Input: part model. Units: mm. Frame: model coordinates. A direction names the side the tool comes from. Round coordinates to 2 decimals unless told otherwise and drop trailing zeros. Write each loop counter-clockwise with the first axis right and the second up, starting at its lowest first coordinate (ties: lowest second). Pieces come first, ordered by that corner, then holes. Notation, with made-up numbers: (39, -30.5) - (91, -30.5) arc R27 cw to (91, -10.5) - close; hole circle Ø5 at (-27.75, 43). An arc over 180 degrees is marked (long way). One line per item, written item: value. Start each with the question number.
```python
from build123d import *

# Parameters (mm, degrees)
BOSS_EXTRUDE1_DEPTH = 10
CUT_EXTRUDE1_REACH  = 52.249
SKETCH3_R           = 3.6
CUT_EXTRUDE3_REACH  = 55.449
CUT_EXTRUDE3_START  = -3.2
SKETCH3_4_R         = 5.5
SKETCH3_4_R_2       = 3.6
CUT_EXTRUDE2_REACH  = 52.249
SKETCH4_R           = 3.6
CUT_EXTRUDE4_START  = -3.2
SKETCH4_3_R         = 5.5
SKETCH4_3_R_2       = 3.6
CUT_EXTRUDE4_DEPTH  = 38.6


with BuildPart() as part:
    # Sketch2 → Boss-Extrude1 (new, symmetric)
    with BuildSketch(Plane(origin=(0, 0, 0), x_dir=(1, 0, 0), z_dir=(0, 1, 0))):
        Polygon((0, 0), (0, 20), (1, 20), (20, 1), (25, 1), (44, 20), (45, 20), (45, 0), (25, 0), (20, 0), align=None)
    extrude(amount=BOSS_EXTRUDE1_DEPTH, both=True)

    # Cut-Extrude1: up to this face of the body (flat: up to its plane)
    cut_extrude1_end = Plane(part.part.faces().sort_by_distance((0.5, 0, -20))[0])
    # Sketch3 → Cut-Extrude1 (cut, up to the picked face)
    with BuildSketch(Plane.XY, mode=Mode.PRIVATE) as cut_extrude1_sk1:
        with Locations((10, 0)):
            Circle(SKETCH3_R)
    cut_extrude1_tool1 = split(extrude(cut_extrude1_sk1.sketch, amount=-CUT_EXTRUDE1_REACH, mode=Mode.PRIVATE), bisect_by=cut_extrude1_end, keep=Keep.BOTH, mode=Mode.PRIVATE)
    # Sketch3 → Cut-Extrude1 (cut, up to the picked face)
    with BuildSketch(Plane.XY, mode=Mode.PRIVATE) as cut_extrude1_sk2:
        with Locations(Location((35, 0, 0), (0, 0, 180))):
            Circle(SKETCH3_R)
    cut_extrude1_tool2 = split(extrude(cut_extrude1_sk2.sketch, amount=-CUT_EXTRUDE1_REACH, mode=Mode.PRIVATE), bisect_by=cut_extrude1_end, keep=Keep.BOTH, mode=Mode.PRIVATE)
    add(cut_extrude1_tool1.solids().sort_by(Axis((10, 0, 0), (0, 0, -1)))[0], mode=Mode.SUBTRACT)
    add(cut_extrude1_tool2.solids().sort_by(Axis((35, 0, 0), (0, 0, -1)))[0], mode=Mode.SUBTRACT)

    # Cut-Extrude3: up to this face of the body (flat: up to its plane)
    cut_extrude3_end = Plane(part.part.faces().sort_by_distance((0.5, 0, -20))[0])
    # Sketch3<4> → Cut-Extrude3 (cut, up to the picked face)
    with BuildSketch(Plane.XY.offset(CUT_EXTRUDE3_START), mode=Mode.PRIVATE) as cut_extrude3_sk1:
        with Locations((10, 0)):
            Circle(SKETCH3_4_R)
        with Locations((10, 0)):
            Circle(SKETCH3_4_R_2, mode=Mode.SUBTRACT)
    cut_extrude3_tool1 = split(extrude(cut_extrude3_sk1.sketch, amount=-CUT_EXTRUDE3_REACH, mode=Mode.PRIVATE), bisect_by=cut_extrude3_end, keep=Keep.BOTH, mode=Mode.PRIVATE)
    # Sketch3<4> → Cut-Extrude3 (cut, up to the picked face)
    with BuildSketch(Plane.XY.offset(CUT_EXTRUDE3_START), mode=Mode.PRIVATE) as cut_extrude3_sk2:
        with Locations(Location((35, 0, 0), (0, 0, 180))):
            Circle(SKETCH3_4_R)
        with Locations((35, 0)):
            Circle(SKETCH3_4_R_2, mode=Mode.SUBTRACT)
    cut_extrude3_tool2 = split(extrude(cut_extrude3_sk2.sketch, amount=-CUT_EXTRUDE3_REACH, mode=Mode.PRIVATE), bisect_by=cut_extrude3_end, keep=Keep.BOTH, mode=Mode.PRIVATE)
    add(cut_extrude3_tool1.solids().sort_by(Axis((4.655563, 0, -3.2), (0, 0, -1)))[0], mode=Mode.SUBTRACT)
    add(cut_extrude3_tool2.solids().sort_by(Axis((40.344437, 0, -3.2), (0, 0, -1)))[0], mode=Mode.SUBTRACT)

    # Cut-Extrude2: up to this face of the body (flat: up to its plane)
    cut_extrude2_end = Plane(part.part.faces().sort_by_distance((45, 0, -10))[0])
    # Sketch4 → Cut-Extrude2 (cut, up to the picked face)
    with BuildSketch(Plane.ZY, mode=Mode.PRIVATE) as cut_extrude2_sk1:
        with Locations((-10, 0)):
            Circle(SKETCH4_R)
    cut_extrude2_tool1 = split(extrude(cut_extrude2_sk1.sketch, amount=-CUT_EXTRUDE2_REACH, mode=Mode.PRIVATE), bisect_by=cut_extrude2_end, keep=Keep.BOTH, mode=Mode.PRIVATE)
    add(cut_extrude2_tool1.solids().sort_by(Axis((0, 0, -10), (1, 0, 0)))[0], mode=Mode.SUBTRACT)

    # Sketch4<3> → Cut-Extrude4 (cut)
    with BuildSketch(Plane.ZY.offset(CUT_EXTRUDE4_START)):
        with Locations((-10, 0)):
            Circle(SKETCH4_3_R)
        with Locations((-10, 0)):
            Circle(SKETCH4_3_R_2, mode=Mode.SUBTRACT)
    extrude(amount=-CUT_EXTRUDE4_DEPTH, mode=Mode.SUBTRACT)


solid = part.part
```
Q1. Cut plane B-B, the plane x = 4. Output: boundary loops of the cut face in (y, z), and give its area (3 significant figures).
Q2. Cut plane C-C, the plane x = 13. Output: boundary loops of the cut face in (y, z), and give its area (3 significant figures).
Q3. Pull-direction query (Y, two-part tool) for faces 1 (the flat face through (0, 0, -14)), 2 (the cylindrical face through (39.86, 3.72, -14.05)), 3 (the flat face through (28, 10, -3)); classes: pulls with the +Y half, pulls with the -Y half, needs draft (parallel to the pull), parting line crosses it, or undercut.
Q4. Cut plane D-D, the plane y = 8.75. Output: boundary loops of the cut face in (x, z), and give its area (3 significant figures).
Q5. Cut plane A-A, the plane z = -1.75. Output: boundary loops of the cut face in (x, y).
Q6. Contact query for flat-ended pins moving along their axis: pin 1 Ø5.5 at (x, y) = (33.5, -1) entering from -Z; pin 2 Ø3 at (x, y) = (14, 3.5) entering from -Z; pin 3 Ø2.5 at (x, y) = (22.5, 1.5) entering from -Z. Output: stop coordinate, or through.
Q7. Access query for faces 4 (the flat face through (44.5, 0.1, -20)), 5 (the cylindrical face through (5.04, 3.72, -14.05)), 6 (the cylindrical face through (13.434, 1.081, -1.578)), 7 (the flat face through (22, 0, -1)), 8 (the flat face through (31, 1, -3.2)). Directions: +Z, -Z, +X, -X, +Y, -Y. A direction counts if a zero-diameter tool reaches every point of the face in a straight line with its end or side. Return the directions, or none.
Q8. Material intervals for probe 1 along Y at (x, z) = (10, -4.5); probe 2 along X at (y, z) = (4, -8.5); probe 3 along X at (y, z) = (-1.75, -3), sorted ascending. Write a range as from..to.
A:
1. outline: (-10, -17) - (10, -17) - (10, 0) - (-10, 0) - close; hole circle Ø11 at (0, -10)
1. area: 245 mm²
2. outline: (-10, -8) - (-5.12, -8) arc R5.5 cw to (-4.61, -7) - (-4.61, -3.2) - (-1.99, -3.2) - (-1.99, 0) - (-10, 0) - close; (1.99, -3.2) - (4.61, -3.2) - (4.61, -7) arc R5.5 cw to (5.12, -8) - (10, -8) - (10, 0) - (1.99, 0) - close
2. area: 102 mm²
3. face 1: needs draft
3. face 2: undercut
3. face 3: pulls with the +Y half
4. outline: (0, -20) - (1, -20) - (20, -1) - (25, -1) - (44, -20) - (45, -20) - (45, 0) - (0, 0) - close
4. area: 444 mm²
5. outline: (0, -10) - (19.25, -10) - (19.25, 10) - (0, 10) - close; (25.75, -10) - (45, -10) - (45, 10) - (25.75, 10) - close; hole circle Ø7.2 at (10, 0); hole circle Ø7.2 at (35, 0)
6. pin 1: stops at z = -3.2
6. pin 2: stops at z = -7.52
6. pin 3: stops at z = -1
7. face 4: -Z, +X, -X, +Y, -Y
7. face 5: none
7. face 6: +Z, -Z
7. face 7: -Z, +Y, -Y
7. face 8: -Z
8. probe 1: y = -10..-5.5, 5.5..10
8. probe 2: x = 0..3.2, 41.8..45
8. probe 3: x = 0..6.85, 13.15..18, 27..31.85, 38.15..45
